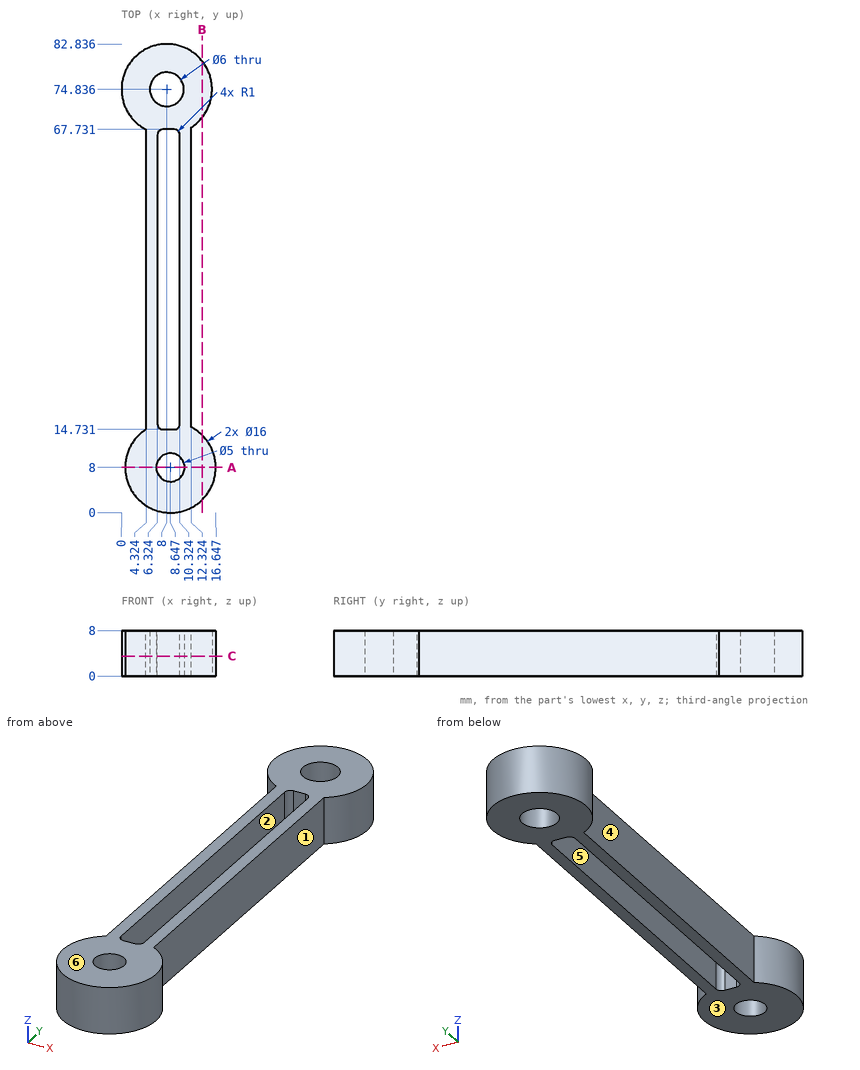
Part print with two shaded views. Sizes in mm from the minimum x, y, z corner. A direction names the side the tool comes from. Coordinates: 2 decimals unless noted, no trailing zeros. Order: outer loops, then holes, each group sorted by start corner. A loop starts at its lowest first (then second) coordinate and runs counter-clockwise, first axis right, second up. Notation, with made-up numbers: M 34.5,21.25 L 78.5,21.25 A23 cw 78.5,38.25 Z; hole C 55,28.5 d2. An arc over 180 degrees is marked long. One line per question, with ' | ' between items. Start each with the question number.
1. Wall check: line 1 along X through (y, z) = (33.5, 3.5); line 2 along Y through (x, z) = (8, 3.5) (1 decimal); line 3 along Y through (x, z) = (8.5, 3.25) (1 decimal). Give the ranges that are in metal, low to high. Write a range as [from, to].
2. Mould opens along Y. For the marked faces 5 and 6 say: +Y half, -Y half, draft (parallel to the pull), parting line (faces both ways), or undercut.
3. Flat gauge pins, fed straight in: P1, Ø2, axis at x = 3, z = 6, coming from the +Y side (1 decimal); P2, Ø1.5, axis at x = 7, z = 6, coming from the +Y side; P3, Ø6, axis at x = 2, y = 12, coming from the -Z side; P4, Ø1, axis at x = 8, z = 3.5, coming from the -Y side. Where does each tip first touch, or does it go through?
4. Cut at B-B (x = 14.25). Write the cut outline in (y, z).
5. Cut at A-A (y = 8). Write the cut outline in (x, z).
6. Cut at C-C (z = 3.5). Write the cut outline in (x, y) (1 decimal).
7. Tool access for the marked faces 1, 2, 3 and 4: list every direction of +Z, -Z, +X, -X, +Y, -Y with a clear straight run to the whole face (end or side of a thin tool).
The answers:
1) line 1: x = [4.32, 6.32], [10.32, 12.32] | line 2: y = [0, 5.6], [10.4, 14.7], [67.7, 71.8], [77.8, 82.8] | line 3: y = [0, 5.5], [10.5, 14.7], [67.7, 71.9], [77.8, 82.8]
2) face 5: undercut | face 6: draft
3) P1: stops at y = 81.8 | P2: stops at y = 82.83 | P3: stops at z = 0 | P4: stops at y = 0
4) outline: M 2.29,0 L 13.71,0 L 13.71,8 L 2.29,8 Z; M 69.84,0 L 79.83,0 L 79.83,8 L 69.84,8 Z
5) outline: M 0.65,0 L 6.15,0 L 6.15,8 L 0.65,8 Z; M 11.15,0 L 16.65,0 L 16.65,8 L 11.15,8 Z
6) outline: M 4.3,14.7 A8 ccw long 12.3,15.1 L 12.3,68.1 A8 ccw long 4.3,67.7 Z; hole C 8,74.8 d6; hole C 8.6,8 d5; hole M 6.3,15.7 A1 ccw 7.3,14.7 L 9.3,14.7 A1 ccw 10.3,15.7 L 10.3,66.7 A1 ccw 9.3,67.7 L 7.3,67.7 A1 ccw 6.3,66.7 Z
7) face 1: +Z, -Z, +X | face 2: +Z, -Z | face 3: -Z, +X, -X, +Y, -Y | face 4: +Z, -Z, -X
